For this review, take the finished solid that the model builds, in its own axes (mm). A direction names the side the tool comes from. Give positions to 0.01 mm unless a question says otherwise; leave off trailing zeros. Order: outer loops, then holes, each group sorted by start corner. A loop starts at its lowest first (then second) coordinate and runs counter-clockwise, first axis right, second up. Notation, with made-up numbers: (-35, 30.25) - (-11, 30.25) arc R26 ccw to (-11, 53.25) - close; hole circle Ø5 at (70.25, -3.5). An arc over 180 degrees is marked (long way). Answer as a JSON object with one key per item and string values. Group by question number.
from build123d import *

# Parameters (mm, degrees)
SKETCH1_W                = 50
SKETCH1_H                = 25
SKETCH1_R                = 4.5
SKETCH1_R_2              = 1.3
BOSS_EXTRUDE2_DEPTH      = 2.5
SKETCH5_W                = 50
SKETCH5_H                = 12
BOSS_EXTRUDE3_DEPTH      = 1.5
SKETCH6_W                = 50
SKETCH6_H                = 26.5
BOSS_EXTRUDE4_DEPTH      = 1.5
SKETCH7_R                = 1.3
CUT_EXTRUDE3_DEPTH       = 23
SKETCH8_R                = 1.6
BOSS_EXTRUDE5_DEPTH      = 4
SKETCH8_3_R              = 8
CUT_EXTRUDE4_DEPTH       = 5
SKETCH9_W                = 24.55
SKETCH9_H                = 21.7
CUT_EXTRUDE5_DEPTH       = 3.8
BOSS_EXTRUDE6_DEPTH      = 22.95
BOSS_EXTRUDE7_DEPTH      = 2
SKETCH8_4_R              = 1.6
CUT_EXTRUDE6_DEPTH       = 5
SKETCH12_W               = 7
SKETCH12_H               = 21
BOSS_EXTRUDE8_DEPTH      = 7.8
SKETCH13_W               = 0.7
SKETCH13_H               = 9
CUT_EXTRUDE7_DEPTH       = 50.95
CUT_EXTRUDE7_DEPTH_BACK  = 26
SKETCH14_W               = 26.5
SKETCH14_H               = 8.5
CUT_EXTRUDE8_DEPTH       = 50.95
CUT_EXTRUDE8_DEPTH_BACK  = 26
SKETCH15_R               = 3
CUT_EXTRUDE9_DEPTH       = 1
CUT_EXTRUDE9_DEPTH_BACK  = 3
SKETCH8_5_R              = 1.6
CUT_EXTRUDE10_DEPTH      = 5
CUT_EXTRUDE10_DEPTH_BACK = 6
SKETCH16_W               = 16.3
SKETCH16_H               = 5
CUT_EXTRUDE11_DEPTH      = 3.2
SKETCH17_R               = 1.45
CUT_EXTRUDE12_DEPTH      = 13.2
SKETCH18_R               = 1.6
CUT_EXTRUDE13_DEPTH      = 3.2
SKETCH19_W               = 17.95
SKETCH19_H               = 5
CUT_EXTRUDE14_DEPTH      = 33.2
BOSS_EXTRUDE9_DEPTH      = 2
SKETCH21_W               = 1.5
SKETCH21_H               = 5
BOSS_EXTRUDE10_DEPTH     = 32.05
SKETCH23_W               = 0.2
SKETCH23_H               = 3.8
CUT_EXTRUDE15_DEPTH      = 42.95
SKETCH17_2_R             = 1.45
CUT_EXTRUDE16_DEPTH      = 20


with BuildPart() as part:
    # Sketch1 → Boss-Extrude2 (new body, symmetric)
    with BuildSketch(Plane(origin=(0, 0, 0), x_dir=(1, 0, 0), z_dir=(0, 1, 0))):
        Rectangle(SKETCH1_W, SKETCH1_H)
        with Locations((11.25, 0)):
            Circle(SKETCH1_R, mode=Mode.SUBTRACT)
        with Locations((-11.25, 0)):
            Circle(SKETCH1_R_2, mode=Mode.SUBTRACT)
    extrude(amount=BOSS_EXTRUDE2_DEPTH, both=True)

    # Sketch5 → Boss-Extrude3 (add, symmetric)
    with BuildSketch(Plane.XY.offset(12.5)):
        with Locations((0, 3.5)):
            Rectangle(SKETCH5_W, SKETCH5_H)
    extrude(amount=BOSS_EXTRUDE3_DEPTH, both=True)

    # Sketch6 → Boss-Extrude4 (add, symmetric)
    with BuildSketch(Plane(origin=(0, 9.5, 0), x_dir=(1, 0, 0), z_dir=(0, 1, 0))):
        with Locations((0, -0.75)):
            Rectangle(SKETCH6_W, SKETCH6_H)
    extrude(amount=BOSS_EXTRUDE4_DEPTH, both=True)

    # Sketch7 → Cut-Extrude3 (cut)
    with BuildSketch(Plane(origin=(0, 11, 0), x_dir=(1, 0, 0), z_dir=(0, 1, 0))):
        with Locations((-11.25, 0)):
            Circle(SKETCH7_R)
        with Locations((11.25, 0)):
            Circle(SKETCH7_R)
    extrude(amount=-CUT_EXTRUDE3_DEPTH, mode=Mode.SUBTRACT)

    # Sketch8 → Boss-Extrude5 (add)
    with BuildSketch(Plane.XZ.offset(2.5)):
        Polygon((47.95, 14.7), (-5.05, 14.7), (-5.05, 14), (25, 14), (25, 9.2), (42.45, 9.2), (42.45, -13.3), (0.45, -13.3), (0.45, -12.5), (-5.05, -12.5), (-5.05, -17.8), (47.95, -17.8), align=None)
        with Locations((45.75, -6.5)):
            Circle(SKETCH8_R, mode=Mode.SUBTRACT)
        with Locations((45.75, 2.4)):
            Circle(SKETCH8_R, mode=Mode.SUBTRACT)
        Polygon((25, 14), (-5.05, 14), (-5.05, -12.5), (0.45, -12.5), (0.45, 9.2), (25, 9.2), align=None)
        with Locations((-2.85, -6.5)):
            Circle(SKETCH8_R, mode=Mode.SUBTRACT)
        with Locations((-2.85, 2.4)):
            Circle(SKETCH8_R, mode=Mode.SUBTRACT)
    extrude(amount=BOSS_EXTRUDE5_DEPTH)

    # Sketch8<3> → Cut-Extrude4 (cut)
    with BuildSketch(Plane.XZ.offset(2.5)):
        with Locations((11.25, 0)):
            Circle(SKETCH8_3_R)
    extrude(amount=-CUT_EXTRUDE4_DEPTH, mode=Mode.SUBTRACT)

    # Sketch9 → Cut-Extrude5 (cut)
    with BuildSketch(Plane.XZ.offset(2.5)):
        with Locations((12.725, -1.65)):
            Rectangle(SKETCH9_W, SKETCH9_H)
    extrude(amount=-CUT_EXTRUDE5_DEPTH, mode=Mode.SUBTRACT)

    # Sketch10 → Boss-Extrude6 (add)
    with BuildSketch(Plane(origin=(25, 0, 0), x_dir=(0, 0, -1), z_dir=(1, 0, 0))):
        Polygon((-14.7, -2.5), (-14.7, 2.5), (14, 2.5), (14, -2.5), (12.3, -2.5), (12.3, 1.3), (-9.2, 1.3), (-9.2, -2.5), align=None)
    extrude(amount=BOSS_EXTRUDE6_DEPTH)

    # Sketch11 → Boss-Extrude7 (add)
    with BuildSketch(Plane(origin=(47.95, 0, 0), x_dir=(0, 0, -1), z_dir=(1, 0, 0))):
        Polygon((-14.7, 2.5), (14, 2.5), (14, -2.5), (17.8, -2.5), (17.8, -6.5), (-14.7, -6.5), align=None)
    extrude(amount=BOSS_EXTRUDE7_DEPTH)

    # Sketch8<4> → Cut-Extrude6 (cut)
    with BuildSketch(Plane.XZ.offset(2.5)):
        with Locations((45.75, -6.5)):
            Circle(SKETCH8_4_R)
        with Locations((45.75, 2.4)):
            Circle(SKETCH8_4_R)
        with Locations((-2.85, -6.5)):
            Circle(SKETCH8_4_R)
        with Locations((-2.85, 2.4)):
            Circle(SKETCH8_4_R)
    extrude(amount=-CUT_EXTRUDE6_DEPTH, mode=Mode.SUBTRACT)

    # Sketch12 → Boss-Extrude8 (add)
    with BuildSketch(Plane.XZ.offset(-1.3)):
        with Locations((46.45, -1.8)):
            Rectangle(SKETCH12_W, SKETCH12_H)
    extrude(amount=BOSS_EXTRUDE8_DEPTH)

    # Sketch13 → Cut-Extrude7 (cut, two sides)
    with BuildSketch(Plane(origin=(0, 0, 0), x_dir=(0, 0, -1), z_dir=(1, 0, 0))) as cut_extrude7_sk:
        with Locations((-14.35, -2)):
            Rectangle(SKETCH13_W, SKETCH13_H)
    extrude(amount=CUT_EXTRUDE7_DEPTH, mode=Mode.SUBTRACT)
    extrude(cut_extrude7_sk.sketch, amount=-CUT_EXTRUDE7_DEPTH_BACK, mode=Mode.SUBTRACT)

    # Sketch14 → Cut-Extrude8 (cut, two sides)
    with BuildSketch(Plane(origin=(0, 0, 0), x_dir=(0, 0, -1), z_dir=(1, 0, 0))) as cut_extrude8_sk:
        with Locations((-0.75, 6.75)):
            Rectangle(SKETCH14_W, SKETCH14_H)
    extrude(amount=CUT_EXTRUDE8_DEPTH, mode=Mode.SUBTRACT)
    extrude(cut_extrude8_sk.sketch, amount=-CUT_EXTRUDE8_DEPTH_BACK, mode=Mode.SUBTRACT)

    # Sketch15 → Cut-Extrude9 (cut, two sides)
    with BuildSketch(Plane(origin=(0, 2.5, 0), x_dir=(1, 0, 0), z_dir=(0, 1, 0))) as cut_extrude9_sk:
        with Locations((-2.85, 6.5)):
            Circle(SKETCH15_R)
        with Locations((-2.85, -2.4)):
            Circle(SKETCH15_R)
        with Locations((45.75, 6.5)):
            Circle(SKETCH15_R)
        with Locations((45.75, -2.4)):
            Circle(SKETCH15_R)
    extrude(amount=CUT_EXTRUDE9_DEPTH, mode=Mode.SUBTRACT)
    extrude(cut_extrude9_sk.sketch, amount=-CUT_EXTRUDE9_DEPTH_BACK, mode=Mode.SUBTRACT)

    # Sketch8<5> → Cut-Extrude10 (cut, two sides)
    with BuildSketch(Plane.XZ.offset(2.5)) as cut_extrude10_sk:
        with Locations((45.75, -6.5)):
            Circle(SKETCH8_5_R)
        with Locations((45.75, 2.4)):
            Circle(SKETCH8_5_R)
    extrude(amount=CUT_EXTRUDE10_DEPTH, mode=Mode.SUBTRACT)
    extrude(cut_extrude10_sk.sketch, amount=-CUT_EXTRUDE10_DEPTH_BACK, mode=Mode.SUBTRACT)

    # Sketch16 → Cut-Extrude11 (cut)
    with BuildSketch(Plane.XY.offset(14)):
        with Locations((8.9, 0)):
            Rectangle(SKETCH16_W, SKETCH16_H)
        with Locations((31, 0)):
            Rectangle(SKETCH16_W, SKETCH16_H)
    extrude(amount=-CUT_EXTRUDE11_DEPTH, mode=Mode.SUBTRACT)

    # Sketch17 → Cut-Extrude12 (cut)
    with BuildSketch(Plane.XY):
        with Locations((8.95, 0)):
            Circle(SKETCH17_R)
        with Locations((30.95, 0)):
            Circle(SKETCH17_R)
    extrude(amount=CUT_EXTRUDE12_DEPTH, mode=Mode.SUBTRACT)

    # Sketch18 → Cut-Extrude13 (cut)
    with BuildSketch(Plane(origin=(0, 2.5, 0), x_dir=(1, 0, 0), z_dir=(0, 1, 0))):
        with Locations((33.75, 1.5)):
            Circle(SKETCH18_R)
    extrude(amount=-CUT_EXTRUDE13_DEPTH, mode=Mode.SUBTRACT)

    # Sketch19 → Cut-Extrude14 (cut)
    with BuildSketch(Plane.XY.offset(14)):
        with Locations((-16.025, 0)):
            Rectangle(SKETCH19_W, SKETCH19_H)
    extrude(amount=-CUT_EXTRUDE14_DEPTH, mode=Mode.SUBTRACT)

    # Sketch20 → Boss-Extrude9 (add)
    with BuildSketch(Plane.XY.offset(14)):
        Polygon((-7.05, 2.5), (49.95, 2.5), (49.95, -6.5), (-5.05, -6.5), (-5.05, -2.5), (-7.05, -2.5), align=None)
    extrude(amount=BOSS_EXTRUDE9_DEPTH)

    # Sketch21 → Boss-Extrude10 (add)
    with BuildSketch(Plane.ZY.offset(-25)):
        with Locations((-13.25, 0)):
            Rectangle(SKETCH21_W, SKETCH21_H)
    extrude(amount=BOSS_EXTRUDE10_DEPTH)

    # Sketch23 → Cut-Extrude15 (cut)
    with BuildSketch(Plane(origin=(0, 0, 0), x_dir=(0, 0, -1), z_dir=(1, 0, 0))):
        with Locations((12.4, -0.6)):
            Rectangle(SKETCH23_W, SKETCH23_H)
    extrude(amount=CUT_EXTRUDE15_DEPTH, mode=Mode.SUBTRACT)

    # Sketch17<2> → Cut-Extrude16 (cut)
    with BuildSketch(Plane.XY):
        with Locations((8.95, 0)):
            Circle(SKETCH17_2_R)
        with Locations((30.95, 0)):
            Circle(SKETCH17_2_R)
    extrude(amount=CUT_EXTRUDE16_DEPTH, mode=Mode.SUBTRACT)


solid = part.part
1) Consider section B-B (z = 2.4). Give the number of separate pieces and of enclosed holes in the cut face, plus the area to 3 significant figures.
2) For pin 1 (1.9 mm diameter, centred on x = 28, z = -16.5, fed in from +Y); pin 2 (3 mm diameter, centred on x = 46.5, z = 1.5, fed in from +Y); pin 3 (1.2 mm diameter, centred on y = -5, z = 0, fed in from -X), all flat-tipped, find the tip position at first contact; note any pin that passes through.
3) For faces 5 (the face through (31.056, 1.446, 7.375)), 6 (the face through (31, 2, 14)), 7 (the face through (42.45, -4, -2)), list the 3-axis set-ups (+Z, -Z, +X, -X, +Y, -Y) from which the entire face can be reached by the end or side of a thin tool; tool diameter is ignored.
4) Mouldability with a two-part tool opening along Z and no side actions: class faces 1 (the face through (31, 2, 10.8)), 2 (the face through (22, -2, 16)), 3 (the face through (46.49, -3.54, 0.98)), 4 (the face through (-6, -2.5, 1)) as released by +Z, released by -Z, zero draft, split by the parting line, or undercut.
5) Consider section D-D (y = -5.5). Give the boundary of the cut face in (x, z), plus the area to 3 significant figures.
6) Consider section A-A (x = 11.25). Give the boundary of the cut face in (y, z), plus the area to 3 significant figures.
7) Consider section C-C (x = 30.95). Give the boundary of the cut face in (y, z), plus the area to 3 significant figures.
8) For line 1 (Z direction, x = -2.85, y = 1.6); line 2 (Z direction, x = 33.75, y = 1.65); line 3 (X direction, y = 0, z = 14.95), list the stretches that pass through material, from the lowest coordinate up.
Result set:
{
 "1": {"separate pieces": "5", "enclosed holes": "0", "area": "83.0 mm2"},
 "2": {"pin 1": "stops at y = -2.5", "pin 2": "stops at y = -0.5", "pin 3": "stops at x = -5.05"},
 "3": {"face 5": "+Z", "face 6": "+Y", "face 7": "-Y"},
 "4": {"face 1": "undercut", "face 2": "released by +Z", "face 3": "undercut", "face 4": "zero draft"},
 "5": {"outline": "(-5.05, -17.8) - (49.95, -17.8) - (49.95, 16) - (-5.05, 16) - close; hole circle Ø3.2 at (-2.85, -6.5); hole circle Ø3.2 at (-2.85, 2.4); hole (0.45, -13.3) - (42.45, -13.3) - (42.45, 9.2) - (0.45, 9.2) - close; hole circle Ø3.2 at (45.75, -6.5); hole circle Ø3.2 at (45.75, 2.4)", "area": "882 mm2"},
 "6": {"outline": "(-6.5, -17.8) - (-2.5, -17.8) - (-2.5, -14) - (2.5, -14) - (2.5, -8) - (1.3, -8) - (1.3, -12.5) - (-2.5, -12.5) - (-2.5, -13.3) - (-6.5, -13.3) - close; (-6.5, 9.2) - (1.3, 9.2) - (1.3, 8) - (2.5, 8) - (2.5, 10.8) - (-2.5, 10.8) - (-2.5, 14) - (2.5, 14) - (2.5, 16) - (-6.5, 16) - close", "area": "77.5 mm2"},
 "7": {"outline": "(-6.5, -17.8) - (-2.5, -17.8) - (-2.5, -14) - (2.5, -14) - (2.5, 10.8) - (1.45, 10.8) - (1.45, 0) - (1.3, 0) - (1.3, -12.5) - (-2.5, -12.5) - (-2.5, -13.3) - (-6.5, -13.3) - close; (-6.5, 9.2) - (-1.45, 9.2) - (-1.45, 10.8) - (-2.5, 10.8) - (-2.5, 14) - (-1.45, 14) - (-1.45, 16) - (-6.5, 16) - close; (1.45, 14) - (2.5, 14) - (2.5, 16) - (1.45, 16) - close", "area": "84.9 mm2"},
 "8": {"line 1": "z = -14 to -9.5, -3.5 to -0.6, 5.4 to 16", "line 2": "z = -14 to -3.1, 0.1 to 10.8, 14 to 16", "line 3": "x = -7.05 to 7.5, 10.4 to 29.5, 32.4 to 49.95"}
}
